from build123d import *

# Parameters (mm, degrees)
EXTRUDE_1_DEPTH          = 15
CUT_EXTRUDE_1_DEPTH      = 15
SKETCH_3_W               = 3
SKETCH_3_H               = 3
EXTRUDE_2_DEPTH          = 0.68
EXTRUDE_3_DEPTH          = 1
EXTRUDE_3_DEPTH_BACK     = 4
CUT_EXTRUDE_2_DEPTH      = 3
CUT_EXTRUDE_2_DEPTH_BACK = 5
FILLET_3_R               = 0.2
FILLET_4_R               = 0.1


with BuildPart() as part:
    # 草图1 → 凸台-拉伸1 (new body)
    with BuildSketch(Plane.XY):
        Polygon((-3.75, 0), (-2.02443152, 15), (2.02443152, 15), (3.75, 0), align=None)
    extrude(amount=EXTRUDE_1_DEPTH)

    # 草图2 → 切除-拉伸1 (cut)
    with BuildSketch(Plane.XY.offset(15)):
        with BuildLine():
            Line((2.715789487, 8.990172149), (3.058642033, 6.009827851))
            Line((3.058642033, 6.009827851), (2.38595414, 5.93244325))
            ThreePointArc((2.38595414, 5.93244325), (-1.086576637, 7.042863273), (2.043101594, 8.912787547))
            Line((2.043101594, 8.912787547), (2.715789487, 8.990172149))
        make_face()
    extrude(amount=-CUT_EXTRUDE_1_DEPTH, mode=Mode.SUBTRACT)

    # 草图3 → 凸台-拉伸2 (add)
    with BuildSketch(Plane(origin=(-3.701021722, 0.425757762, 0), x_dir=(0, 0, 1), z_dir=(-0.9934480991964022, 0.11428418177094966, 0))):
        with Locations((7.5, 7.120897653)):
            Rectangle(SKETCH_3_W, SKETCH_3_H)
    extrude(amount=EXTRUDE_2_DEPTH)

    # 草图4 → 凸台-拉伸3 (add, two sides: drawn at the far end of the back side and taken through both)
    with BuildSketch(Plane(origin=(0, 0, 6), x_dir=(-1, 0, 0), z_dir=(0, 0, -1)).offset(-EXTRUDE_3_DEPTH_BACK)):
        with BuildLine():
            Line((5.593690162, 5.848486661), (4.65546812, 5.740555569))
            ThreePointArc((4.65546812, 5.740555569), (4.17347222, 5.855308115), (3.734476016, 6.085026481))
            Line((3.734476016, 6.085026481), (3.391044919, 9.070400006))
            ThreePointArc((3.391044919, 9.070400006), (3.76641144, 9.393800948), (4.209759811, 9.615003156))
            Line((4.209759811, 9.615003156), (5.147981853, 9.722934248))
            Line((5.147981853, 9.722934248), (5.593690162, 5.848486661))
        make_face()
    extrude(amount=EXTRUDE_3_DEPTH + EXTRUDE_3_DEPTH_BACK)

    # 草图5 → 切除-拉伸2 (cut, two sides: drawn at the far end of the back side and taken through both)
    with BuildSketch(Plane(origin=(0.642379689, 5.584070089, 0), x_dir=(0.9934480991964022, -0.11428418177094966, 0), z_dir=(-0.11428418177094966, -0.9934480991964022, 0)).offset(-CUT_EXTRUDE_2_DEPTH_BACK)):
        with BuildLine():
            Line((-6.225430372, 9.45), (-6.225430372, 10))
            Line((-6.225430372, 10), (-4.405430372, 10))
            Line((-4.405430372, 10), (-4.405430372, 9.002531198))
            ThreePointArc((-4.405430372, 9.002531198), (-4.815297141, 9.280914794), (-5.281020651, 9.45))
            Line((-5.281020651, 9.45), (-6.225430372, 9.45))
        make_face()
        with BuildLine():
            Line((-6.225430372, 5.55), (-5.281020651, 5.55))
            ThreePointArc((-5.281020651, 5.55), (-4.815297141, 5.719085206), (-4.405430372, 5.997468802))
            Line((-4.405430372, 5.997468802), (-4.405430372, 5))
            Line((-4.405430372, 5), (-6.225430372, 5))
            Line((-6.225430372, 5), (-6.225430372, 5.55))
        make_face()
    extrude(amount=CUT_EXTRUDE_2_DEPTH + CUT_EXTRUDE_2_DEPTH_BACK, mode=Mode.SUBTRACT)

    # 圆角3
    fillet_3_edges = [part.edges().sort_by_distance(p)[0] for p in [
        (0, 0, 15),
        (3.404321016, 3.004913926, 15),
        (2.370110504, 11.995086074, 0),
        (2.370110504, 11.995086074, 15),
        (3.058642033, 6.009827851, 7.5),
        (2.715789487, 8.990172149, 7.5),
        (0, 15, 15),
        (3.404321016, 3.004913926, 0),
        (0, 0, 0),
        (-2.88721576, 7.5, 0),
        (0, 15, 0),
        (-2.88721576, 7.5, 15),
        (2.02443152, 15, 7.5),
        (3.75, 0, 7.5),
        (-3.75, 0, 7.5),
        (-2.02443152, 15, 7.5),
    ]]
    fillet(fillet_3_edges, radius=FILLET_3_R)

    # 圆角4
    fillet_4_edges = [part.edges().sort_by_distance(p)[0] for p in [
        (-5.593690162, 5.848486661, 7.5),
        (-5.147981853, 9.722934248, 7.5),
        (-5.370836008, 7.785710454, 9.45),
        (-5.370836008, 7.785710454, 5.55),
    ]]
    fillet(fillet_4_edges, radius=FILLET_4_R)


solid = part.part
Verification items for the finished model (mm, model axes). A direction names the side the tool comes from. Give positions to 0.01 mm unless a question says otherwise; leave off trailing zeros. Loops run counter-clockwise (first coordinate to the right, second up) from the corner with the lowest first, then second, coordinate; pieces in that order, holes last.
1. Tool access check on faces 5 (the cylindrical face through (-4, 7.7, 9.3)), 6 (the flat face through (-5, 8, 5.55)), 7 (the flat face through (-3, 8, 6)). Record the directions out of +Z, -Z, +X, -X, +Y, -Y that give a thin tool (end or side, any length) a straight path to the whole face; none if there is none.
Derived:
face 5: +Z
face 6: -Z, -X, +Y, -Y
face 7: -Z
2. Cross-section at A-A on x = 1. Record the cut outline in (y, z).
Derived:
outline: (0, 0.2) arc R0.2 ccw to (0.2, 0) - (5.27, 0) - (5.27, 15) - (0.2, 15) arc R0.2 ccw to (0, 14.8) - close; (9.27, 0) - (14.8, 0) arc R0.2 ccw to (15, 0.2) - (15, 14.8) arc R0.2 ccw to (14.8, 15) - (9.27, 15) - close
3. Release check for a two-part mould opening along X. For faces 1 (the flat face through (-5.37, 7.81, 7.53)), 2 (the flat face through (-5, 8, 9.45)), 3 (the flat face through (-3, 8, 9)), 4 (the cylindrical face through (2.33, 11.86, 0.06)) record: +X half, -X half, draft (parallel to the pull), parting line (faces both ways), or undercut.
Derived:
face 1: -X half
face 2: draft
face 3: undercut
face 4: +X half
4. Cross-section at B-B on z = 14.25. Record the cut outline in (x, y).
Derived:
outline: (-3.72, 0.22) arc R0.2 ccw to (-3.53, 0) - (3.53, 0) arc R0.2 ccw to (3.72, 0.22) - (3.08, 5.81) arc R0.2 ccw to (2.86, 5.99) - (2.39, 5.93) arc R2 cw (long way) to (2.04, 8.91) - (2.52, 8.97) arc R0.2 ccw to (2.69, 9.19) - (2.04, 14.82) arc R0.2 ccw to (1.85, 15) - (-1.85, 15) arc R0.2 ccw to (-2.04, 14.82) - close
5. Go/stop test with flat-tipped pins: P1, Ø0.8, axis at x = -3.5, y = 7.5, coming from the -Z side; P2, Ø1.4, axis at x = -5, y = 7.5, coming from the +Z side; P3, Ø5, axis at y = 13.5, z = 4.5, coming from the -X side. Record where each tip stops, or that it passes through.
Derived:
P1: stops at z = 5.76
P2: stops at z = 9.45
P3: stops at x = -2.48
6. Material ranges on probe 1 along Y at (x, z) = (3, 2); probe 2 along Z at (x, y) = (-3.25, 6.75); probe 3 along Y at (x, z) = (-0.75, 2.25), recorded low to high.
Derived:
probe 1: y = 0 to 5.95
probe 2: z = 6 to 9
probe 3: y = 0 to 6.14, 8.4 to 15
